```python
from build123d import *

# Parameters (mm, degrees)
SKETCH_W     = 13.1
SKETCH_H     = 5.05
PAD_DEPTH    = 8
CHAMFER_SIZE = 0.3


with BuildPart() as part:
    # Sketch → Pad (new body)
    with BuildSketch(Plane.XY):
        Polygon((-8.95, 3.225), (-8.95, -3.225), (-2.25, -3.225), (-2.25, -4.425), (2.25, -4.425), (2.25, -3.225), (8.95, -3.225), (8.95, 3.225), align=None)
        Rectangle(SKETCH_W, SKETCH_H, mode=Mode.SUBTRACT)
    extrude(amount=PAD_DEPTH)

    # Chamfer
    chamfer_edges = [part.edges().sort_by_distance(p)[0] for p in [
        (6.55, 0, 8),
        (0, 2.525, 8),
        (-6.55, 0, 8),
        (0, -2.525, 8),
    ]]
    chamfer(chamfer_edges, length=CHAMFER_SIZE)


solid = part.part
```
Could you check a few things on this model? Use its own coordinates, in mm. A direction names the side the tool comes from. Round coordinates to 2 decimals unless told otherwise and drop trailing zeros. Loops run counter-clockwise (first coordinate to the right, second up) from the corner with the lowest first, then second, coordinate; pieces in that order, holes last.
Q1. I want a section at B-B (y = -0.5). Write out the boundary of the cut face in (x, z).
Q2. Please list where these lines run through material, in increasing order: L1, parallel to Y at x = -1.25, z = 3.75 (3 decimals); L2, parallel to Y at x = 6, z = 4.5 (3 decimals); L3, parallel to X at y = -1.5, z = 1.25.
Q3. Thinking about a two-plate mould opening in X: for faces 4 (the flat face through (0, -2.525, 4)), 5 (the flat face through (0, -3, 8)), 6 (the flat face through (8.95, 0, 4)), 7 (the flat face through (0, 2.525, 4)), which applies, pulls with the +X half, pulls with the -X half, needs draft (parallel to the pull), parting line crosses it, or undercut?
Q4. I want a section at A-A (x = 0.5). Write out the boundary of the cut face in (y, z) (3 decimals).
Q5. For P1, Ø1.3, axis at y = -3.5, z = 5, coming from the +X side; P2, Ø2, axis at x = 7, z = 5, coming from the -Y side (3 decimals), each with a flat end and sliding along its axis, tell me the tip position at first contact or that it passes through.
Q6. On a 3-axis mill with a long thin cutter (end or side, diameter ignored), from which of +Z, -Z, +X, -X, +Y, -Y can I reach the whole of each face in a straight line? I mean faces 1 (the flat face through (-6.55, 0, 4)), 2 (the flat face through (-2.25, -4, 4)), 3 (the flat face through (2.25, -4, 4)). Say none if no direction works.
Q7. I want a section at D-D (y = -3.5). Write out the boundary of the cut face in (x, z), and give its area (3 significant figures).
Q8. I want a section at C-C (z = 1.5). Write out the boundary of the cut face in (x, y) (3 decimals), and give its area (3 significant figures).
Answer below:
1. outline: (-8.95, 0) - (-6.55, 0) - (-6.55, 7.7) - (-6.85, 8) - (-8.95, 8) - close; (6.55, 0) - (8.95, 0) - (8.95, 8) - (6.85, 8) - (6.55, 7.7) - close
2. L1: y = -4.425 to -2.525, 2.525 to 3.225
2. L2: y = -3.225 to -2.525, 2.525 to 3.225
2. L3: x = -8.95 to -6.55, 6.55 to 8.95
3. face 4: undercut
3. face 5: needs draft
3. face 6: pulls with the +X half
3. face 7: undercut
4. outline: (-4.425, 0) - (-2.525, 0) - (-2.525, 7.7) - (-2.825, 8) - (-4.425, 8) - close; (2.525, 0) - (3.225, 0) - (3.225, 8) - (2.825, 8) - (2.525, 7.7) - close
5. P1: stops at x = 8.95
5. P2: stops at y = -3.225
6. face 1: +Z, -Z
6. face 2: +Z, -Z, -X, -Y
6. face 3: +Z, -Z, +X, -Y
7. outline: (-2.25, 0) - (2.25, 0) - (2.25, 8) - (-2.25, 8) - close
7. area: 36.0 mm2
8. outline: (-8.95, -3.225) - (-2.25, -3.225) - (-2.25, -4.425) - (2.25, -4.425) - (2.25, -3.225) - (8.95, -3.225) - (8.95, 3.225) - (-8.95, 3.225) - close; hole (-6.55, -2.525) - (6.55, -2.525) - (6.55, 2.525) - (-6.55, 2.525) - close
8. area: 54.7 mm2
